from build123d import *

# Parameters (mm, degrees)
SKETCH1_W           = 46.097722286
SKETCH1_H           = 46.097722286
BOSS_EXTRUDE1_DEPTH = 32.5
SKETCH2_W           = 46.097722286
SKETCH2_H           = 39.997722286
BOSS_EXTRUDE2_DEPTH = 27.5


with BuildPart() as part:
    # Sketch1 → Boss-Extrude1 (new body)
    with BuildSketch(Plane(origin=(0, 0, 0), x_dir=(-1, 0, 0), z_dir=(0, 0, 1))):
        Rectangle(SKETCH1_W, SKETCH1_H)
    extrude(amount=-BOSS_EXTRUDE1_DEPTH)

    # Sketch2 → Boss-Extrude2 (add)
    with BuildSketch(Plane(origin=(0, 0, -32.5), x_dir=(-1, 0, 0), z_dir=(0, 0, -1))):
        Rectangle(SKETCH2_W, SKETCH2_H)
    extrude(amount=BOSS_EXTRUDE2_DEPTH)


solid = part.part
Model file for the job. Use its own axes, mm. A direction names the side the tool comes from. Give positions to 0.01 mm unless a question says otherwise; leave off trailing zeros. Write each loop counter-clockwise with the first axis right and the second up, starting at its lowest first coordinate (ties: lowest second). Pieces come first, ordered by that corner, then holes. Notation, with made-up numbers: M 47.5,77 L 102.5,77 A27 cw 102.5,102 Z; hole C 18,66.25 d3. An arc over 180 degrees is marked long. One line per item, written item: value. Start each with the question number.
Q1. 3-axis set-ups, long thin cutter, end or side, ignore diameter. For faces 1 (the flat face through (0, 22, -32.5)), 2 (the flat face through (-23.049, 0, -30)), 3 (the flat face through (0, -19.999, -46)): which of +Z, -Z, +X, -X, +Y, -Y reach the whole face in a straight line?
Q2. Probe probe 1 along Y at (x, z) = (10, -46.5). List the from-to ranges inside material, lowest first. Write a range as [from, to].
Q3. Drop flat-ended pins along their axis: pin 1 Ø22 at (x, z) = (7, -49) entering from -Y; pin 2 Ø14 at (x, z) = (10.5, -51) entering from +Y; pin 3 Ø2.5 at (x, y) = (-4.5, -21.5) entering from -Z. Give the stop position or say it passes through.
Q4. Saw through at B-B, the plane z = -53.5. Write the cut outline in (x, y).
Q5. Saw through at A-A, the plane x = -13.5. Write the cut outline in (y, z), plus the area to 3 significant figures.
Output values:
1. face 1: -Z, +X, -X, +Y
1. face 2: +Z, -Z, -X, +Y, -Y
1. face 3: -Z, +X, -X, -Y
2. probe 1: y = [-20, 20]
3. pin 1: stops at y = -20
3. pin 2: stops at y = 20
3. pin 3: stops at z = -32.5
4. outline: M -23.05,-20 L 23.05,-20 L 23.05,20 L -23.05,20 Z
5. outline: M -23.05,-32.5 L -20,-32.5 L -20,-60 L 20,-60 L 20,-32.5 L 23.05,-32.5 L 23.05,0 L -23.05,0 Z
5. area: 2,600 mm²
